```python
from build123d import *

# Parameters (mm, degrees)
BOSS_EXTRUDE1_DEPTH     = 5
BOSS_EXTRUDE2_DEPTH     = 3
BOSS_EXTRUDE3_DEPTH     = 3
SKETCH10_W              = 9.5
SKETCH10_H              = 5
BOSS_EXTRUDE4_DEPTH     = 15.78
SKETCH11_W              = 9.5
SKETCH11_H              = 2
BOSS_EXTRUDE5_DEPTH     = 40
BOSS_EXTRUDE6_DEPTH     = 6.09393
SKETCH14_R              = 1.8
CUT_EXTRUDE1_DEPTH      = 6.3
SKETCH15_W              = 51.153217575
SKETCH15_H              = 86.05062267
CUT_EXTRUDE3_DEPTH      = 6
CUT_EXTRUDE3_DEPTH_BACK = 19.78
SKETCH16_W              = 9.603970124
SKETCH16_H              = 11.884913028
CUT_EXTRUDE4_DEPTH      = 17.733728816


with BuildPart() as part:
    # Sketch3 → Revolve1 (revolve)
    with BuildSketch(Plane.XY):
        Polygon((-62.694264441, 11.733728816), (-64.884531744, 11.733728816), (-64.884531744, 5.639799249), (-60.884531744, 5.639799249), (-60.884531744, 6.650679103), (-62.884531744, 6.650679103), (-62.884531744, 10.250679103), (-60.884531744, 10.250679103), (-60.884531744, 11.733728816), align=None)
    revolve(axis=Axis((-49.744264441, 0, 0), (0, 1, 0)))

    # Sketch7 → Boss-Extrude1 (add)
    with BuildSketch(Plane(origin=(0, 11.733728816, 0), x_dir=(1, 0, 0), z_dir=(0, 1, 0))):
        with BuildLine():
            Line((-50.244264441, 15.132008921), (-50.244264441, 13.130751112))
            ThreePointArc((-50.244264441, 13.130751112), (-49.744264441, 13.140267302), (-49.244264441, 13.130751112))
            Line((-49.244264441, 13.130751112), (-49.244264441, 15.132008921))
            ThreePointArc((-49.244264441, 15.132008921), (-49.744264441, 15.140267302), (-50.244264441, 15.132008921))
        make_face()
    extrude(amount=BOSS_EXTRUDE1_DEPTH)

    # Sketch8 → Boss-Extrude2 (add)
    with BuildSketch(Plane(origin=(0, 16.733728816, 0), x_dir=(1, 0, 0), z_dir=(0, 1, 0))):
        with BuildLine():
            Line((-50.244264441, 15.132008921), (-50.244264441, 13.130751112))
            Line((-50.244264441, 13.130751112), (-50.244264441, -4.369248888))
            Line((-50.244264441, -4.369248888), (-49.244264441, -4.369248888))
            Line((-49.244264441, -4.369248888), (-49.244264441, 13.130751112))
            Line((-49.244264441, 13.130751112), (-49.244264441, 15.132008921))
            ThreePointArc((-49.244264441, 15.132008921), (-49.744264441, 15.140267302), (-50.244264441, 15.132008921))
        make_face()
    extrude(amount=-BOSS_EXTRUDE2_DEPTH)

    # Sketch9 → Boss-Extrude3 (add)
    with BuildSketch(Plane(origin=(0, 11.733728816, 0), x_dir=(1, 0, 0), z_dir=(0, 1, 0))):
        with BuildLine():
            Line((-54.494264441, 14.375854548), (-54.494264441, 39.375854548))
            Line((-54.494264441, 39.375854548), (-44.994264441, 39.375854548))
            Line((-44.994264441, 39.375854548), (-44.994264441, 14.375854548))
            ThreePointArc((-44.994264441, 14.375854548), (-47.092177082, 14.906177465), (-49.244264441, 15.132008921))
            ThreePointArc((-49.244264441, 15.132008921), (-49.744264441, 15.140267302), (-50.244264441, 15.132008921))
            ThreePointArc((-50.244264441, 15.132008921), (-52.3963518, 14.906177465), (-54.494264441, 14.375854548))
        make_face()
    extrude(amount=-BOSS_EXTRUDE3_DEPTH)

    # Sketch10 → Boss-Extrude4 (add)
    with BuildSketch(Plane.XZ.offset(-8.733728816)):
        with Locations((-49.744264441, -36.875854548)):
            Rectangle(SKETCH10_W, SKETCH10_H)
    extrude(amount=BOSS_EXTRUDE4_DEPTH)

    # Sketch11 → Boss-Extrude5 (add)
    with BuildSketch(Plane(origin=(0, 0, -39.375854548), x_dir=(-1, 0, 0), z_dir=(0, 0, -1))):
        with Locations((49.744264441, -6.046271184)):
            Rectangle(SKETCH11_W, SKETCH11_H)
    extrude(amount=BOSS_EXTRUDE5_DEPTH)

    # Sketch13 → Boss-Extrude6 (add)
    with BuildSketch(Plane(origin=(0, 11.733728816, 0), x_dir=(1, 0, 0), z_dir=(0, 1, 0))):
        with BuildLine():
            Line((-28.603997139, 3.15), (-34.935307895, 3.15))
            ThreePointArc((-34.935307895, 3.15), (-34.603997139, 0), (-34.935307895, -3.15))
            Line((-34.935307895, -3.15), (-28.603997139, -3.15))
            Line((-28.603997139, -3.15), (-28.603997139, 3.15))
        make_face()
        with BuildLine():
            Line((-70.884531744, 3.15), (-70.884531744, -3.15))
            Line((-70.884531744, -3.15), (-64.553220987, -3.15))
            ThreePointArc((-64.553220987, -3.15), (-64.884531744, 0), (-64.553220987, 3.15))
            Line((-64.553220987, 3.15), (-70.884531744, 3.15))
        make_face()
    extrude(amount=-BOSS_EXTRUDE6_DEPTH)

    # Sketch14 → Cut-Extrude1 (cut)
    with BuildSketch(Plane.XY.offset(3.15)):
        with Locations((-31.769652517, 8.686764033)):
            Circle(SKETCH14_R)
        with Locations((-67.718876365, 8.686764033)):
            Circle(SKETCH14_R)
    extrude(amount=-CUT_EXTRUDE1_DEPTH, mode=Mode.SUBTRACT)

    # Sketch15 → Cut-Extrude3 (cut, two sides)
    with BuildSketch(Plane(origin=(0, 11.733728816, 0), x_dir=(1, 0, 0), z_dir=(0, 1, 0))) as cut_extrude3_sk:
        with Locations((-49.018725857, 43.025311335)):
            Rectangle(SKETCH15_W, SKETCH15_H)
    extrude(amount=CUT_EXTRUDE3_DEPTH, mode=Mode.SUBTRACT)
    extrude(cut_extrude3_sk.sketch, amount=-CUT_EXTRUDE3_DEPTH_BACK, mode=Mode.SUBTRACT)

    # Sketch16 → Cut-Extrude4 (cut, through all)
    with BuildSketch(Plane(origin=(0, 0, 0), x_dir=(1, 0, 0), z_dir=(0, 1, 0))):
        with Locations((-50.086315959, -0.525030424)):
            Rectangle(SKETCH16_W, SKETCH16_H)
    extrude(amount=CUT_EXTRUDE4_DEPTH, mode=Mode.SUBTRACT)


solid = part.part
```
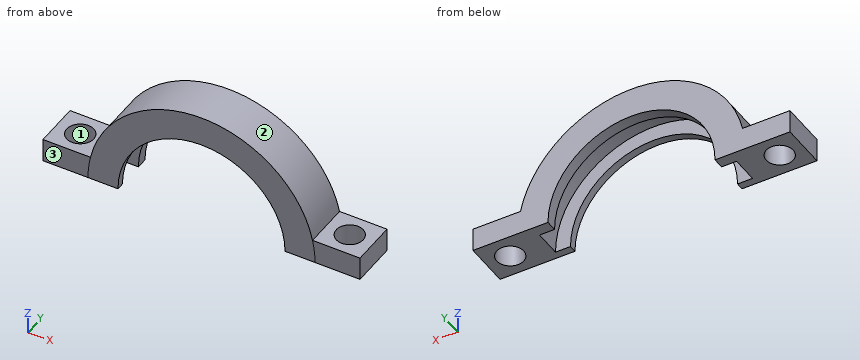
Geometry: final body of the model. Coordinates: model frame, mm. Face numbers are marked on the shaded views. Round coordinates to 2 decimals unless told otherwise and drop trailing zeros. Order: outer loops, then holes, each group sorted by start corner. A loop starts at its lowest first (then second) coordinate and runs counter-clockwise, first axis right, second up. Notation, with made-up numbers: (77.5, -14) -> (117.5, -14) arc R12 cw to (117.5, -5) -> close; hole circle Ø5 at (43, 89.5). An arc over 180 degrees is marked (long way). Use one line per item in the form item = value. Start each with the question number.
1. Line query: probe 1 along X at (y, z) = (9.5, 1); probe 2 along X at (y, z) = (8, 3.25); probe 3 along X at (y, z) = (9.25, 7.25). Output: solid intervals per line, ascending.
2. Draft query along X for the marked faces 1, 2 and 3. Return one class per face: pulls with the +X half, pulls with the -X half, needs draft (parallel to the pull), parting line crosses it, or undercut.
3. Cut plane A-A (z = 1.25). Return the cut outline in (x, y), then the cut area to 3 significant figures.
4. Cut plane B-B (y = 6.25). Return the cut outline in (x, z).
5. Cut plane D-D (x = -67). Return the cut outline in (y, z), then the cut area to 3 significant figures.
6. Cut plane C-C (z = 10.25). Return the cut outline in (x, y).
7. Pin query (flat end, axial travel): pin 1 Ø2 at (x, y) = (-53.5, 7.5) entering from +Z; pin 2 Ø1.8 at (x, y) = (-68.5, 10) entering from +Z; pin 3 Ø2 at (y, z) = (6.5, 4.5) entering from +X; pin 4 Ø5 at (x, z) = (-57.5, 3) entering from +Y. Return the tip coordinate at first contact, or that it passes through.
Solution:
q1.probe_1 = -70.88 to -69.32, -66.11 to -62.85, -36.64 to -33.38, -30.16 to -28.6
q1.probe_2 = -64.53 to -62.48, -37.01 to -34.96
q1.probe_3 = -63.04 to -60.7, -38.79 to -36.45
q2.face_1 = undercut
q2.face_2 = parting line crosses it
q2.face_3 = needs draft
q3.outline = (-70.88, 5.64) -> (-60.81, 5.64) -> (-60.81, 6.65) -> (-62.82, 6.65) -> (-62.82, 10.25) -> (-60.81, 10.25) -> (-60.81, 11.73) -> (-70.88, 11.73) -> close; (-38.67, 5.64) -> (-28.6, 5.64) -> (-28.6, 11.73) -> (-38.67, 11.73) -> (-38.67, 10.25) -> (-36.66, 10.25) -> (-36.66, 6.65) -> (-38.67, 6.65) -> close; hole circle Ø3.6 at (-67.72, 8.69); hole circle Ø3.6 at (-31.77, 8.69)
q3.area = 87.9 mm^2
q4.outline = (-70.88, 0) -> (-60.88, 0) arc R11.14 cw to (-38.6, 0) -> (-28.6, 0) -> (-28.6, 3.15) -> (-34.94, 3.15) arc R15.14 ccw to (-64.55, 3.15) -> (-70.88, 3.15) -> close
q5.outline = (5.64, 0) -> (7.04, 0) -> (7.04, 3.15) -> (5.64, 3.15) -> close; (10.34, 0) -> (11.73, 0) -> (11.73, 3.15) -> (10.34, 3.15) -> close
q5.area = 8.80 mm^2
q6.outline = (-60.89, 5.64) -> (-54.11, 5.64) -> (-54.11, 6.65) -> (-57.97, 6.65) -> (-57.97, 10.25) -> (-54.11, 10.25) -> (-54.11, 11.73) -> (-60.89, 11.73) -> close; (-45.38, 5.64) -> (-38.6, 5.64) -> (-38.6, 11.73) -> (-45.38, 11.73) -> (-45.38, 10.25) -> (-41.52, 10.25) -> (-41.52, 6.65) -> (-45.38, 6.65) -> close
q7.pin_1 = 14.89
q7.pin_2 = 3.15
q7.pin_3 = -35.01
q7.pin_4 = through
